```python
from build123d import *

# Parameters (mm, degrees)
F0_W      = 116.3828
F0_H      = 76.2
F1_DEPTH  = 16.51
F2_R      = 12.7
F3_DEPTH  = 63.5
F4_R      = 12.7
F7_R      = 5.08
F9_DEPTH  = 15.24
F10_R     = 12.7
F11_DEPTH = 12.7
F13_DEPTH = 25.4
F15_DEPTH = 5.08
F16_W     = 47.8547876488
F16_H     = 29.861765301
F17_DEPTH = 5.08


with BuildPart() as f1:
    # F0 (on Top) → F1 (new body)
    with BuildSketch(Plane.XY):
        Rectangle(F0_W, F0_H)
    extrude(amount=-F1_DEPTH)

    # F2 (on Right) → F3 (join, symmetric)
    with BuildSketch(Plane.YZ):
        with Locations((38.1, 0)):
            Circle(F2_R)
    extrude(amount=F3_DEPTH, both=True)

    # F4
    f4_edges = [f1.edges().sort_by_distance(p)[0] for p in [
        (-58.1914, -38.1, -8.255),
        (58.1914, -38.1, -8.255),
    ]]
    fillet(f4_edges, radius=F4_R)

    # F5 (on Top) → F6 (revolve, cut)
    with BuildSketch(Plane.XY):
        Polygon((-63.5, 50.8635), (-63.5, 38.1), (0, 38.1), (63.5, 38.1), (63.5, 50.8635), (29.845, 50.8635), (29.845, 47.9425), (0, 47.9425), (-29.845, 47.9425), (-29.845, 50.8635), align=None)
    revolve(axis=Axis((31.75, 38.1, 0), (1, 0, 0)), mode=Mode.SUBTRACT)

    # F7
    f7_edges = [f1.edges().sort_by_distance(p)[0] for p in [
        (58.1914, 6.35, -16.51),
    ]]
    fillet(f7_edges, radius=F7_R)

    # F8 (on face) → F9 (cut)
    with BuildSketch(Plane.XY):
        with BuildLine():
            Line((55.6514, -23.0505), (55.6514, 23.0505))
            Line((55.6514, 23.0505), (-55.6514, 23.0505))
            Line((-55.6514, 23.0505), (-55.6514, -23.0505))
            Line((-55.6514, -23.0505), (-55.6514, -25.4))
            ThreePointArc((-55.6514, -25.4), (-52.6756048969, -32.5842048969), (-45.4914, -35.56))
            Line((-45.4914, -35.56), (45.4914, -35.56))
            ThreePointArc((45.4914, -35.56), (52.6756048969, -32.5842048969), (55.6514, -25.4))
            Line((55.6514, -25.4), (55.6514, -23.0505))
        make_face()
    extrude(amount=-F9_DEPTH, mode=Mode.SUBTRACT)

    # F10 (on Right) → F11 (cut, symmetric)
    with BuildSketch(Plane.YZ):
        with Locations((38.1, 0)):
            Circle(F10_R)
    extrude(amount=F11_DEPTH, both=True, mode=Mode.SUBTRACT)

    # F12 (on face) → F13 (cut)
    with BuildSketch(Plane.XZ.offset(-23.0505)):
        with BuildLine():
            Line((6.985, -1.605504806), (-6.985, -1.605504806))
            ThreePointArc((-6.985, -1.605504806), (-10.5771024484, -3.0934023576), (-12.065, -6.685504806))
            Line((-12.065, -6.685504806), (-12.065, -8.4159879088))
            ThreePointArc((-12.065, -8.4159879088), (-10.5771024484, -12.0080903572), (-6.985, -13.4959879088))
            Line((-6.985, -13.4959879088), (6.985, -13.4959879088))
            ThreePointArc((6.985, -13.4959879088), (10.5771024484, -12.0080903572), (12.065, -8.4159879088))
            Line((12.065, -8.4159879088), (12.065, -6.685504806))
            ThreePointArc((12.065, -6.685504806), (10.5771024484, -3.0934023576), (6.985, -1.605504806))
        make_face()
    extrude(amount=-F13_DEPTH, mode=Mode.SUBTRACT)

    # F14 (on face) → F15 (join)
    with BuildSketch(Plane.XY.offset(-15.24)):
        Polygon((-41.275, -12.8604971486), (-41.275, 17.78), (-36.195, 17.78), (-36.195, 19.5553619415), (-43.2557910681, 19.5553619415), (-43.2557910681, -12.8604971486), align=None)
        Polygon((36.195, 19.5553619415), (36.195, 17.78), (41.275, 17.78), (41.275, -12.8604971486), (43.2557910681, -12.8604971486), (43.2557910681, 19.5553619415), align=None)
    extrude(amount=F15_DEPTH)

    # F16 (on face) → F17 (cut)
    with BuildSketch(Plane.XY):
        with Locations((-34.2640061756, -23.1691173495)):
            Rectangle(F16_W, F16_H)
        with Locations((34.2640061756, -23.1691173495)):
            Rectangle(F16_W, F16_H)
    extrude(amount=-F17_DEPTH, mode=Mode.SUBTRACT)


solid = f1.part
```
Work out the finished part from the listing and answer in its coordinate system (mm). A direction names the side the tool comes from. Coordinates: 2 decimals unless noted, no trailing zeros. Loops run counter-clockwise (first coordinate to the right, second up) from the corner with the lowest first, then second, coordinate; pieces in that order, holes last. Notation, with made-up numbers: (40.5, 87.25) - (57.5, 87.25) arc R13 ccw to (57.5, 93.25) - close; hole circle Ø9 at (58, 65). An arc over 180 degrees is marked (long way). Use a Markdown table: item, result.
Item 1: Find section A-A, the plane x = -27.5. Determine the outline of the cut face in (y, z) (1 decimal).
Evaluation:
| item | result |
|---|---|
| outline | (-38.1, -11.4) arc R5.1 ccw to (-33, -16.5) - (38.1, -16.5) - (38.1, -12.7) arc R12.7 ccw (long way) to (25.4, 0) - (23.1, 0) - (23.1, -15.2) - (-35.6, -15.2) - (-35.6, -5.1) - (-38.1, -5.1) - close; hole circle Ø19.7 at (38.1, 0) |
Item 2: Find section B-B, the plane z = 2. Determine the outline of the cut face in (x, y) (3 decimals).
Evaluation:
| item | result |
|---|---|
| outline | (-29.845, 25.558) - (-12.7, 25.558) - (-12.7, 28.463) - (-29.845, 28.463) - close; (-29.845, 47.737) - (-12.7, 47.737) - (-12.7, 50.642) - (-29.845, 50.642) - close; (12.7, 25.558) - (29.845, 25.558) - (29.845, 28.463) - (12.7, 28.463) - close; (12.7, 47.737) - (29.845, 47.737) - (29.845, 50.642) - (12.7, 50.642) - close |
Item 3: The mould has two halves that part along X. Classify faces 5 (the cylindrical face through (56.743, 6.794, -14.982)), 6 (the flat face through (-1, -6, -15.24)), 7 (the flat face through (-10.337, -37, -3)), 8 (the cylindrical face through (0.637, -36.651, -14.982)): +X half, -X half, draft (parallel to the pull), parting line (faces both ways), or undercut.
Evaluation:
| item | result |
|---|---|
| face 5 | +X half |
| face 6 | undercut |
| face 7 | -X half |
| face 8 | draft |
Item 4: Given pin 1 Ø10 at (y, z) = (12, 6) entering from -X; pin 2 Ø3 at (y, z) = (-36.5, -2.5) entering from -X; pin 3 Ø10 at (x, y) = (10.5, -9.5) entering from +Z; pin 4 Ø1.5 at (x, z) = (6, -0.5) entering from +Y, each flat-ended and moving along its own axis, determine where each tip first touches the part or whether it passes through.
Evaluation:
| item | result |
|---|---|
| pin 1 | passes through |
| pin 2 | stops at x = -10.34 |
| pin 3 | stops at z = -15.24 |
| pin 4 | stops at y = 25.46 |
Item 5: For faces 1 (the flat face through (-12.7, 41.8, -9.3)), 2 (the flat face through (10.337, -37, -3)), 3 (the flat face through (-5, 24, 0)), 4 (the cylindrical face through (52.6, -32.66, -10.09)), determine the directions among +Z, -Z, +X, -X, +Y, -Y from which every point of the face is accessible in a straight line to the end or side of a thin tool.
Evaluation:
| item | result |
|---|---|
| face 1 | +Z, +Y |
| face 2 | +Z, +X, -Y |
| face 3 | +Z, +X, -X, -Y |
| face 4 | +Z |
Item 6: Find section C-C, the plane y = 2. Determine the outline of the cut face in (x, z) (3 decimals).
Evaluation:
| item | result |
|---|---|
| outline | (-58.191, -11.43) arc R5.08 ccw to (-53.111, -16.51) - (53.111, -16.51) arc R5.08 ccw to (58.191, -11.43) - (58.191, 0) - (55.651, 0) - (55.651, -15.24) - (43.256, -15.24) - (43.256, -10.16) - (41.275, -10.16) - (41.275, -15.24) - (-41.275, -15.24) - (-41.275, -10.16) - (-43.256, -10.16) - (-43.256, -15.24) - (-55.651, -15.24) - (-55.651, 0) - (-58.191, 0) - close |
Item 7: Consider probe 1 along X at (y, z) = (-6, -5); probe 2 along Z at (x, y) = (-16, 38); probe 3 along Z at (x, y) = (-33, -27.5). Determine where each line is inside the solid, lowest interval first. Write a range as from..to.
Evaluation:
| item | result |
|---|---|
| probe 1 | x = -58.19..-55.65, 55.65..58.19 |
| probe 2 | z = -16.51..-9.84, 9.84..12.7 |
| probe 3 | z = -16.51..-15.24 |
Item 8: Find section D-D, the plane y = 35. Determine the outline of the cut face in (x, z) (3 decimals).
Evaluation:
| item | result |
|---|---|
| outline | (-58.102, -12.381) arc R5.08 ccw to (-53.111, -16.51) - (53.111, -16.51) arc R5.08 ccw to (58.102, -12.381) - (29.845, -12.381) - (29.845, -9.342) - (12.7, -9.342) - (12.7, -12.316) - (10.24, -12.316) arc R5.08 cw to (6.985, -13.496) - (-6.985, -13.496) arc R5.08 cw to (-10.24, -12.316) - (-12.7, -12.316) - (-12.7, -9.342) - (-29.845, -9.342) - (-29.845, -12.381) - close; (-29.845, 9.342) - (-12.7, 9.342) - (-12.7, 12.316) - (-29.845, 12.316) - close; (12.7, 9.342) - (29.845, 9.342) - (29.845, 12.316) - (12.7, 12.316) - close |
